Autodesk Inventor part; units mm, degrees
ref_plane "YZ Plane" through (0, 0, 0) normal (1, 0, 0) x (0, 1, 0)
ref_plane "XZ Plane" through (0, 0, 0) normal (0, 1, 0) x (-1, 0, 0)
ref_plane "XY Plane" through (0, 0, 0) normal (0, 0, 1) x (1, 0, 0)
sketch "Sketch1" plane through (0, 0, 0) normal (1, 0, 0) x (0, 1, 0)
  line L0 (0, 0) -> (0, -609.6)
  line L1 (0, -609.6) -> (426.8465, -609.6)
  line L2 (426.8465, -609.6) -> (0, 0)
  line L3 (25.4, -80.5585) -> (378.0536, -584.2)
  line L4 (378.0536, -584.2) -> (25.4, -584.2)
  line L5 (25.4, -584.2) -> (25.4, -80.5585)
  dimension "d0" = 609.6
  dimension "d1" = 35
  dimension "d2" = 25.4
  dimension "d3" = 25.4
  dimension "d4" = 25.4
extrude "Extrusion1" add sketch "Sketch1" along normal mid plane 25.4
sketch "Sketch2" plane through (12.7, 0, 0) normal (1, 0, 0) x (0, 0, -1)
  line L0 (0, 0) -> (609.6, 0)
  line L1 (0, 0) -> (653.0822, 457.2931)
  line L2 (80.5585, 25.4) -> (584.2, 378.0536)
  line L3 (79.2672, 24.4958) -> (584.2, 378.0536)
  line L4 (584.2, 378.0536) -> (657.7963, 429.5863)
  line L5 (584.2, 25.4) -> (80.5585, 25.4)
  line L6 (80.5585, 25.4) -> (44.2835, 0)
  line L7 (44.2835, 0) -> (0, 0)
  line L8 (609.6, 0) -> (609.6, 426.8465)
  line L9 (609.6, 426.8465) -> (609.6, 393.6892)
  point P0 (609.6, 511.5151)
  point P1 (68.5783, 24.3867)
  point P2 (69.7859, 25.4)
properties part number "ballRampLeftSideV04-30-60"
Work out the finished part from the listing and answer in its coordinate system (mm). A direction names the side the tool comes from. Coordinates: 2 decimals unless noted, no trailing zeros. Loops run counter-clockwise (first coordinate to the right, second up) from the corner with the lowest first, then second, coordinate; pieces in that order, holes last. Notation, with made-up numbers: (79, -31.75) -> (94, -31.75) arc R23 cw to (94, -13.75) -> close; hole circle Ø2 at (83, 42.25). An arc over 180 degrees is marked (long way). Answer as CSV lines item,"result".
Q1. Each of these flat-tipped pins is pushed along its axis until it touches: pin 1 (2 mm diameter, centred on x = -8, y = 382.5, fed in from +Z); pin 2 (5 mm diameter, centred on x = -3.5, z = -315.5, fed in from +Y); pin 3 (8 mm diameter, centred on x = -9, z = -294.5, fed in from +Y). Where does it stop, or does it pass through?
Findings:
pin 1,"stops at z = -544.84"
pin 2,"stops at y = 222.67"
pin 3,"stops at y = 209.01"
Q2. A tool of negligible diameter and unlimited length cuts with its end or side. For faces 1 (the face through (12.7, 23, -394)), 2 (the face through (0, 204, -584.2)), from which of +Z, -Z, +X, -X, +Y, -Y can it reach the whole face along a straight path? Write none if from no direction.
Findings:
face 1,"+Z, -Z, +X, +Y, -Y"
face 2,"+X, -X"
Q3. For a pull along Z with two mould halves and no side action, classify faces 3 (the face through (0, 25.4, -336)), 4 (the face through (0, 0, -301)), 5 (the face through (-0.178, 199.258, -328.854)), 6 (the face through (-0.178, 216.411, -309.067)) as +Z half, -Z half, draft (parallel to the pull), parting line (faces both ways), or undercut.
Findings:
face 3,"undercut"
face 4,"draft"
face 5,"undercut"
face 6,"+Z half"
Q4. Find the intervals of material crossed by probe 1 along Z at (x, y) = (0.5, 355); probe 2 along Y at (x, z) = (-4, -194); probe 3 along Z at (x, y) = (5, 105), in increasing order.
Findings:
probe 1,"z = -609.6 to -584.2, -551.28 to -506.99"
probe 2,"y = 0 to 25.4, 104.83 to 135.84"
probe 3,"z = -609.6 to -584.2, -194.24 to -149.96"
Q5. The part is cut by section A-A on z = -142.5. Write down the section's boundary in (x, y).
Findings:
outline,"(-12.7, 0) -> (12.7, 0) -> (12.7, 25.4) -> (-12.7, 25.4) -> close; (-12.7, 68.77) -> (12.7, 68.77) -> (12.7, 99.78) -> (-12.7, 99.78) -> close"
Q6. The part is cut by section B-B on x = -8.25. Write down the section's boundary in (y, z), and give its area (3 significant figures).
Findings:
outline,"(0, -609.6) -> (426.85, -609.6) -> (0, 0) -> close; hole (25.4, -584.2) -> (378.05, -584.2) -> (25.4, -80.56) -> close"
area,"41,300 mm²"
Q7. The part is cut by section C-C on y = 111. Write down the section's boundary in (x, z).
Findings:
outline,"(-12.7, -609.6) -> (12.7, -609.6) -> (12.7, -584.2) -> (-12.7, -584.2) -> close; (-12.7, -202.81) -> (12.7, -202.81) -> (12.7, -158.52) -> (-12.7, -158.52) -> close"
